from build123d import *

# Parameters (mm, degrees)
F0_R     = 26.123678
F1_DEPTH = 93.77381
F2_R     = 8.171962
F3_DEPTH = 107.8945
F4_W     = 52.7304
F4_H     = 52.288964
F5_DEPTH = 4.39529


with BuildPart() as f1:
    # F0 (on Front) → F1 (new body)
    with BuildSketch(Plane.XZ):
        Circle(F0_R)
    extrude(amount=F1_DEPTH)

    # F2 (on face) → F3 (join)
    with BuildSketch(Plane(origin=(0, 0, 0), x_dir=(-1, 0, 0), z_dir=(0, 1, 0))):
        Circle(F2_R)
    extrude(amount=F3_DEPTH)

    # F4 (on face) → F5 (join)
    with BuildSketch(Plane(origin=(0, 107.8945, 0), x_dir=(-1, 0, 0), z_dir=(0, 1, 0))):
        Rectangle(F4_W, F4_H)
    extrude(amount=F5_DEPTH)


solid = f1.part
CAD build for the part. Positions are in the model's coordinates, mm. A direction names the side the tool comes from. Give positions to 0.01 mm unless a question says otherwise; leave off trailing zeros. Loops run counter-clockwise (first coordinate to the right, second up) from the corner with the lowest first, then second, coordinate; pieces in that order, holes last. Notation, with made-up numbers: M -38,43 L 3,43 A11 ccw 3,55 Z; hole C 55,56 d2. An arc over 180 degrees is marked long. One line per question, with ' | ' between items. Start each with the question number.
1. Flat gauge pins, fed straight in: pin 1 (10 mm diameter, centred on y = -25, z = -19, fed in from -X); pin 2 (12 mm diameter, centred on x = -12, y = -33, fed in from +Z); pin 3 (1 mm diameter, centred on x = -18.5, y = -15, fed in from +Z). Where does each tip first touch, or does it go through?
2. Saw through at A-A on z = 14. Give the cut face in (x, y).
3. Saw through at B-B on x = 0. Give the cut face in (y, z).
4. Saw through at C-C on z = 0. Give the cut face in (x, y).
5. Probe L1, parallel to Y at x = -5, z = 24.5; L2, parallel to Y at x = 24.5, z = -20; L3, parallel to Z at x = -5, y = 30. List the from-to ranges inside material, lowest first. Write a range as from..to.
6. Saw through at D-D on y = -76. Give the cut face in (x, z), plus the area to 3 significant figures.
7. 3-axis set-ups, long thin cutter, end or side, ignore diameter. For faces 1 (the face through (-3.77, 53.19, -7.25)), 2 (the face through (14.04, -46.23, 22.03)), 3 (the face through (0, 110, 26.144)): which of +Z, -Z, +X, -X, +Y, -Y reach the whole face in a straight line?
Result sheet:
1) pin 1: stops at x = -22.06 | pin 2: stops at z = 25.43 | pin 3: stops at z = 18.93
2) outline: M -26.37,107.89 L 26.37,107.89 L 26.37,112.29 L -26.37,112.29 Z; M -22.06,-93.77 L 22.06,-93.77 L 22.06,0 L -22.06,0 Z
3) outline: M -93.77,-26.12 L 0,-26.12 L 0,-8.17 L 107.89,-8.17 L 107.89,-26.14 L 112.29,-26.14 L 112.29,26.14 L 107.89,26.14 L 107.89,8.17 L 0,8.17 L 0,26.12 L -93.77,26.12 Z
4) outline: M -26.37,107.89 L -8.17,107.89 L -8.17,0 L -26.12,0 L -26.12,-93.77 L 26.12,-93.77 L 26.12,0 L 8.17,0 L 8.17,107.89 L 26.37,107.89 L 26.37,112.29 L -26.37,112.29 Z
5) L1: y = -93.77..0, 107.89..112.29 | L2: y = 107.89..112.29 | L3: z = -6.46..6.46
6) outline: C 0,0 d52.25 | area: 2,140 mm^2
7) face 1: none | face 2: -Y | face 3: +Z, +X, -X, +Y, -Y
